Verification items for the finished model (mm, model axes). A direction names the side the tool comes from. Give positions to 0.01 mm unless a question says otherwise; leave off trailing zeros. Loops run counter-clockwise (first coordinate to the right, second up) from the corner with the lowest first, then second, coordinate; pieces in that order, holes last. Notation, with made-up numbers: M -36,-10 L -8,-10 A23 cw -8,7 Z; hole C 19,50 d6. An arc over 180 degrees is marked long. Answer in a Markdown table with one row per item.
Autodesk Fusion 360 part; units mm, degrees
sketch "Sketch1" plane through (0, 0, 0) normal (1, 0, 0) x (0, 1, 0)
  line L0 (0, 0) -> (0, 12.5)
  line L1 (0, 12.5) -> (25, 12.5)
  line L2 (25, 12.5) -> (25, 10)
  line L3 (25, 10) -> (45, 10)
  line L4 (45, 10) -> (45, 12.5)
  line L5 (45, 12.5) -> (66, 12.5) construction
  line L6 (66, 12.5) -> (66, 11)
  line L7 (45, 12.5) -> (66, 11)
  line L8 (66, 12.5) -> (66, 13.5)
  line L9 (66, 13.5) -> (92, 13.5) construction
  line L10 (92, 13.5) -> (92, 8.5) construction
  line L11 (66, 13.5) -> (92, 8.5)
  line L12 (66, 13.5) -> (98, 13.5) construction
  line L13 (98, 13.5) -> (98, 0)
  arc A0 (98, 1.2362) -> (92, 8.5) centre (90.6031, 1.2362) ccw
  line L14 (98, 0) -> (0, 0)
  dimension "d1" = 12.5
  dimension "d2" = 25
  dimension "d4" = 20
  dimension "d6" = 21
  dimension "d9" = 26
  dimension "d10" = 5
  dimension "d11" = 13.5
  dimension "d12" = 12.5
  dimension "d13" = 10
  dimension "d14" = 11
  dimension "d15" = 32
  dimension "d16" = 7.3969
revolve "Revolve1" add sketch "Sketch1" angle 360 about axis through (0, 98, 0) along (0, -1, 0)
hole "Hole1" at (0, 0, 0) direction (0, 1, 0) diameter 11.6675 depth 12 tip angle 118
chamfer "Chamfer1" distance 10 distance2 2 1 edges at (-11.6541, 0, 4.5202) measured on face at (1.2446, 16.6667, 12.4379)
equation "d1 = 25 mm / 2"
Item 1: Go/stop test with flat-tipped pins: pin 1 (1.5 mm diameter, centred on x = 2, z = 3, fed in from -Y); pin 2 (6 mm diameter, centred on y = 28.5, z = 9, fed in from -X); pin 3 (9.5 mm diameter, centred on x = 0, z = 0, fed in from -Y). Record where each tip stops, or that it passes through.
Reported:
| item | result |
|---|---|
| pin 1 | stops at y = 12.89 |
| pin 2 | stops at x = -8 |
| pin 3 | stops at y = 12.65 |
Item 2: Scan lines: L1, parallel to X at y = 2.5, z = 0; L2, parallel to Z at x = -5.5, y = 54; L3, parallel to X at y = 4, z = -1. Record each from-to range of solid material in increasing order. Write a range as [from, to].
Reported:
| item | result |
|---|---|
| L1 | x = [-11, -5.83], [5.83, 11] |
| L2 | z = [-10.5, 10.5] |
| L3 | x = [-11.26, -5.75], [5.75, 11.26] |
Item 3: Tool access check on faces 4 (the cylindrical face through (-9.76, 35.14, -2.17)), 5 (the conical face through (6.4, 81.7, -8.3)), 6 (the cylindrical face through (3.755, 17.605, 11.923)). Record the directions out of +Z, -Z, +X, -X, +Y, -Y that give a thin tool (end or side, any length) a straight path to the whole face; none if there is none.
Reported:
| item | result |
|---|---|
| face 4 | none |
| face 5 | +Y |
| face 6 | -Y |
Item 4: Sectioned sample at B-B (y = 67). Record the cut outline in (x, z), and give its area (3 significant figures).
Reported:
| item | result |
|---|---|
| outline | C 0,0 d26.62 |
| area | 556 mm^2 |
Item 5: Release check for a two-part mould opening along Y. For faces 1 (the flat face through (10, 66, -5)), 2 (the flat face through (0, 98, 0)), 3 (the conical face through (-6.7, 2.8, -8.8)) record: released by +Y, released by -Y, zero draft, split by the parting line, or undercut.
Reported:
| item | result |
|---|---|
| face 1 | undercut |
| face 2 | released by +Y |
| face 3 | released by -Y |
Item 6: Sectioned sample at A-A (y = 49). Record the cut outline in (x, z), and give its area (3 significant figures).
Reported:
| item | result |
|---|---|
| outline | C 0,0 d24.43 |
| area | 469 mm^2 |
